Design review of the part shown in the three views and the two pictorial views. Dimensions are in mm from the part's minimum x, y and z. Round coordinates to 2 decimals unless told otherwise and drop trailing zeros. Loops run counter-clockwise (first coordinate to the right, second up) from the corner with the lowest first, then second, coordinate; pieces in that order, holes last.
1. Consider section C-C on z = 50.8. State the section outline as (x, y) points (1 decimal).
2. Consider section D-D on z = 12.7. State the section outline as (x, y) points (1 decimal), then the cut area to 3 significant figures.
3. Consider section A-A on x = 38.1. State the section outline as (y, z) points (1 decimal).
4. To check wall thickness, follow line 1 along Z through (x, y) = (12.7, 1.3); line 2 along Z through (x, y) = (38.1, 1.05); line 3 along Z through (x, y) = (28, 2.15). State the ranges of each line that lie inside material, in increasing order.
5. Clearance check with a flat-ended pin moving along its axis: pin 1 Ø1.5 at (x, y) = (43, 2) entering from +Z. State where the tip first meets the part, or that it passes through.
6. Consider section B-B on y = 0.9. State the section outline as (x, z) points.
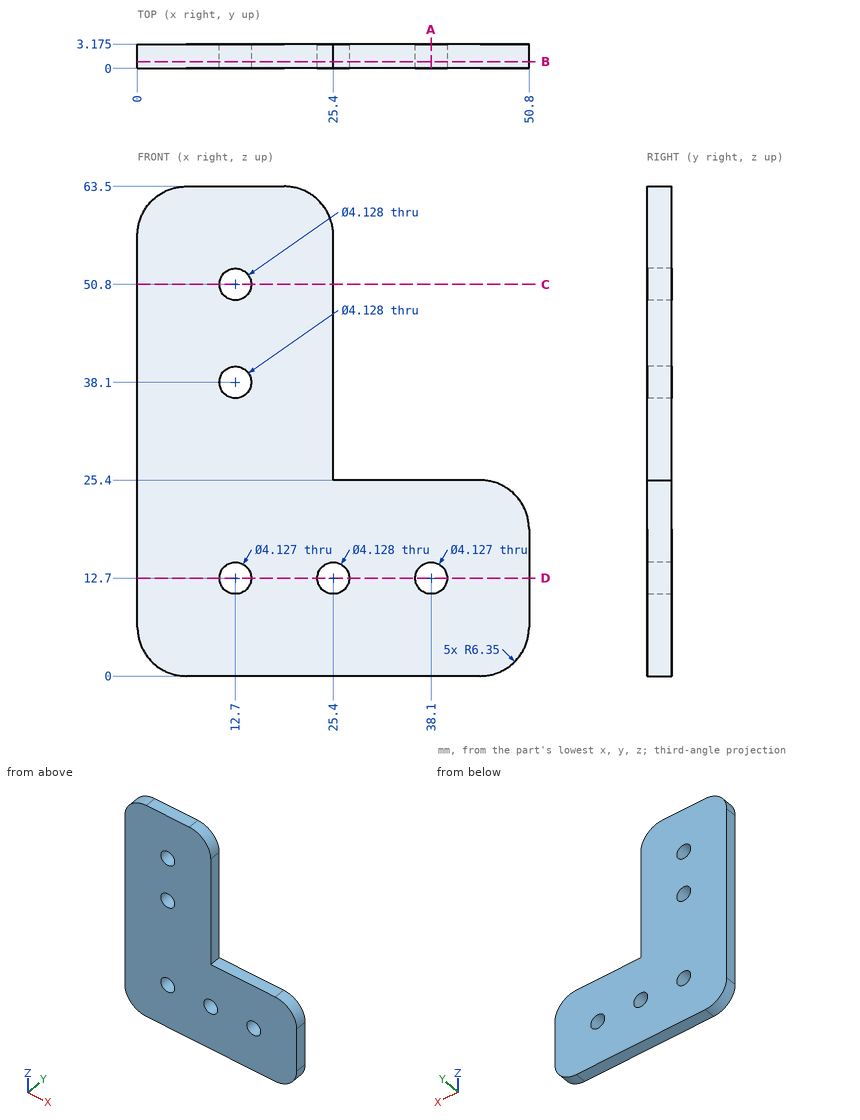
Resolved:
1. outline: (0, 0) - (10.6, 0) - (10.6, 3.2) - (0, 3.2) - close; (14.8, 0) - (25.4, 0) - (25.4, 3.2) - (14.8, 3.2) - close
2. outline: (0, 0) - (10.6, 0) - (10.6, 3.2) - (0, 3.2) - close; (14.8, 0) - (23.3, 0) - (23.3, 3.2) - (14.8, 3.2) - close; (27.5, 0) - (36, 0) - (36, 3.2) - (27.5, 3.2) - close; (40.2, 0) - (50.8, 0) - (50.8, 3.2) - (40.2, 3.2) - close
2. area: 122 mm2
3. outline: (0, 0) - (3.2, 0) - (3.2, 10.6) - (0, 10.6) - close; (0, 14.8) - (3.2, 14.8) - (3.2, 25.4) - (0, 25.4) - close
4. line 1: z = 0 to 10.64, 14.76 to 36.04, 40.16 to 48.74, 52.86 to 63.5
4. line 2: z = 0 to 10.64, 14.76 to 25.4
4. line 3: z = 0 to 25.4
5. pin 1: stops at z = 25.4
6. outline: (0, 6.35) arc R6.35 ccw to (6.35, 0) - (44.45, 0) arc R6.35 ccw to (50.8, 6.35) - (50.8, 19.05) arc R6.35 ccw to (44.45, 25.4) - (25.4, 25.4) - (25.4, 57.15) arc R6.35 ccw to (19.05, 63.5) - (6.35, 63.5) arc R6.35 ccw to (0, 57.15) - close; hole circle Ø4.13 at (12.7, 12.7); hole circle Ø4.13 at (12.7, 38.1); hole circle Ø4.13 at (12.7, 50.8); hole circle Ø4.13 at (25.4, 12.7); hole circle Ø4.13 at (38.1, 12.7)
